from build123d import *

# Parameters (mm, degrees)
F1_DEPTH     = 2
F3_DEPTH     = 25
F4_T1_DEPTH  = 50
F4_T3_DEPTH  = 120
F4_T6_ANGLE  = 90
F4_T8_ANGLE  = 90
F4_T10_ANGLE = 90
F4_T12_ANGLE = 90
F5_R         = 0.5


# Not quite as in the source:
# - a fillet or chamfer that OpenCascade refuses, or shapes differently, is made with other operations: its cross-section is extruded or revolved along the edge and cut away or added


with BuildPart() as f1:
    # F0 (on Front) → F1 (new body)
    with BuildSketch(Plane.XZ):
        with BuildLine():
            ThreePointArc((70, 25), (67.0710678119, 32.0710678119), (60, 35))
            Line((60, 35), (-60, 35))
            ThreePointArc((-60, 35), (-67.0710678119, 32.0710678119), (-70, 25))
            Line((-70, 25), (-70, -25))
            ThreePointArc((-70, -25), (-67.0710678119, -32.0710678119), (-60, -35))
            Line((-60, -35), (60, -35))
            ThreePointArc((60, -35), (67.0710678119, -32.0710678119), (70, -25))
            Line((70, -25), (70, 25))
        make_face()
    extrude(amount=F1_DEPTH)

    # F2 (on Front) → F3 (cut)
    with BuildSketch(Plane.XZ):
        with BuildLine():
            Line((-62, -8), (-62, 8))
            ThreePointArc((-62, 8), (-62.5857864376, 9.4142135624), (-64, 10))
            ThreePointArc((-64, 10), (-65.4142135624, 9.4142135624), (-66, 8))
            Line((-66, 8), (-66, -8))
            ThreePointArc((-66, -8), (-65.4142135624, -9.4142135624), (-64, -10))
            ThreePointArc((-64, -10), (-62.5857864376, -9.4142135624), (-62, -8))
        make_face()
    extrude(amount=F3_DEPTH, mode=Mode.SUBTRACT)

    # F4: fillet of radius 2.5 on 1 edges, made by hand

    # F4_s2 → F4_t1 (cut)
    with BuildSketch(Plane.XY.offset(-25)):
        with BuildLine():
            ThreePointArc((-67.5505102572, -2), (-69.1316490873, -1.4364916731), (-70, 0))
            Line((-70, 0), (-70, -2))
            Line((-70, -2), (-67.5505102572, -2))
        make_face()
        with BuildLine():
            ThreePointArc((70, 0), (69.1316490873, -1.4364916731), (67.5505102572, -2))
            Line((67.5505102572, -2), (70, -2))
            Line((70, -2), (70, 0))
        make_face()
    extrude(amount=F4_T1_DEPTH, mode=Mode.SUBTRACT)

    # F4_s4 → F4_t3 (cut)
    with BuildSketch(Plane.YZ.offset(-60)):
        with BuildLine():
            ThreePointArc((-2, -32.5505102572), (-1.4364916731, -34.1316490873), (0, -35))
            Line((0, -35), (-2, -35))
            Line((-2, -35), (-2, -32.5505102572))
        make_face()
        with BuildLine():
            ThreePointArc((0, 35), (-1.4364916731, 34.1316490873), (-2, 32.5505102572))
            Line((-2, 32.5505102572), (-2, 35))
            Line((-2, 35), (0, 35))
        make_face()
    extrude(amount=F4_T3_DEPTH, mode=Mode.SUBTRACT)

    # F4_s5 → F4_t6 (revolve, cut)
    with BuildSketch(Plane.XY.offset(-25)):
        with BuildLine():
            ThreePointArc((-67.5505102572, -2), (-69.1316490873, -1.4364916731), (-70, 0))
            Line((-70, 0), (-70, -2))
            Line((-70, -2), (-67.5505102572, -2))
        make_face()
    revolve(axis=Axis((-60, -2, -25), (0, -1, 0)), revolution_arc=F4_T6_ANGLE, mode=Mode.SUBTRACT)

    # F4_s7 → F4_t8 (revolve, cut)
    with BuildSketch(Plane.YZ.offset(60)):
        with BuildLine():
            ThreePointArc((-2, -32.5505102572), (-1.4364916731, -34.1316490873), (0, -35))
            Line((0, -35), (-2, -35))
            Line((-2, -35), (-2, -32.5505102572))
        make_face()
    revolve(axis=Axis((60, -2, -25), (0, -1, 0)), revolution_arc=F4_T8_ANGLE, mode=Mode.SUBTRACT)

    # F4_s9 → F4_t10 (revolve, cut)
    with BuildSketch(Plane.XY.offset(25)):
        with BuildLine():
            ThreePointArc((70, 0), (69.1316490873, -1.4364916731), (67.5505102572, -2))
            Line((67.5505102572, -2), (70, -2))
            Line((70, -2), (70, 0))
        make_face()
    revolve(axis=Axis((60, -2, 25), (0, -1, 0)), revolution_arc=F4_T10_ANGLE, mode=Mode.SUBTRACT)

    # F4_s11 → F4_t12 (revolve, cut)
    with BuildSketch(Plane.YZ.offset(-60)):
        with BuildLine():
            ThreePointArc((-2, 32.5505102572), (-1.4364916731, 34.1316490873), (0, 35))
            Line((0, 35), (-2, 35))
            Line((-2, 35), (-2, 32.5505102572))
        make_face()
    revolve(axis=Axis((-60, -2, 25), (0, -1, 0)), revolution_arc=F4_T12_ANGLE, mode=Mode.SUBTRACT)

    # F5
    f5_edges = [f1.edges().sort_by_distance(p)[0] for p in [
        (-62, -2, 0),
        (-64, -2, 10),
        (-66, -2, 0),
        (-64, -2, -10),
    ]]
    fillet(f5_edges, radius=F5_R)


solid = f1.part
Check sheet for the modelled part. Datum: model origin and axes. Units: mm. Round coordinates to 2 decimals unless told otherwise and drop trailing zeros. Loops run counter-clockwise (first coordinate to the right, second up) from the corner with the lowest first, then second, coordinate; pieces in that order, holes last. Notation, with made-up numbers: M 24,8.25 L 66,8.25 A22 ccw 66,42.25 Z; hole C 66,69.5 d6. An arc over 180 degrees is marked long. One line per question, with ' | ' between items. Start each with the question number.
Item 1: Section check B-B (x = -21.5). Record the boundary of the cut face in (y, z).
Item 2: Section check C-C (y = -0.85). Record the boundary of the cut face in (x, z).
Item 3: Scan lines: probe 1 along X at (y, z) = (-1.3, 9); probe 2 along X at (y, z) = (-0.8, -8); probe 3 along X at (y, z) = (-0.6, -19.5). Record each from-to range of solid material in increasing order.
Item 4: Section check A-A (z = -5.5). Record the boundary of the cut face in (x, y), and give its area (3 significant figures).
Worked out:
1) outline: M -2,-32.55 A2.5 ccw 0,-35 L 0,35 A2.5 ccw -2,32.55 Z
2) outline: M -69.65,-25 A9.65 ccw -60,-34.65 L 60,-34.65 A9.65 ccw 69.65,-25 L 69.65,25 A9.65 ccw 60,34.65 L -60,34.65 A9.65 ccw -69.65,25 Z; hole M -66,-8 A2 ccw -62,-8 L -62,8 A2 ccw -66,8 Z
3) probe 1: -69.29 to -65.73, -62.27 to 69.29 | probe 2: -69.69 to -66, -62 to 69.69 | probe 3: -69.8 to 69.8
4) outline: M -70,0 A2.5 ccw -67.55,-2 L -66.5,-2 A0.5 ccw -66,-1.5 L -66,0 Z; M -62,-1.5 A0.5 ccw -61.5,-2 L 67.55,-2 A2.5 ccw 70,0 L -62,0 Z | area: 269 mm^2
